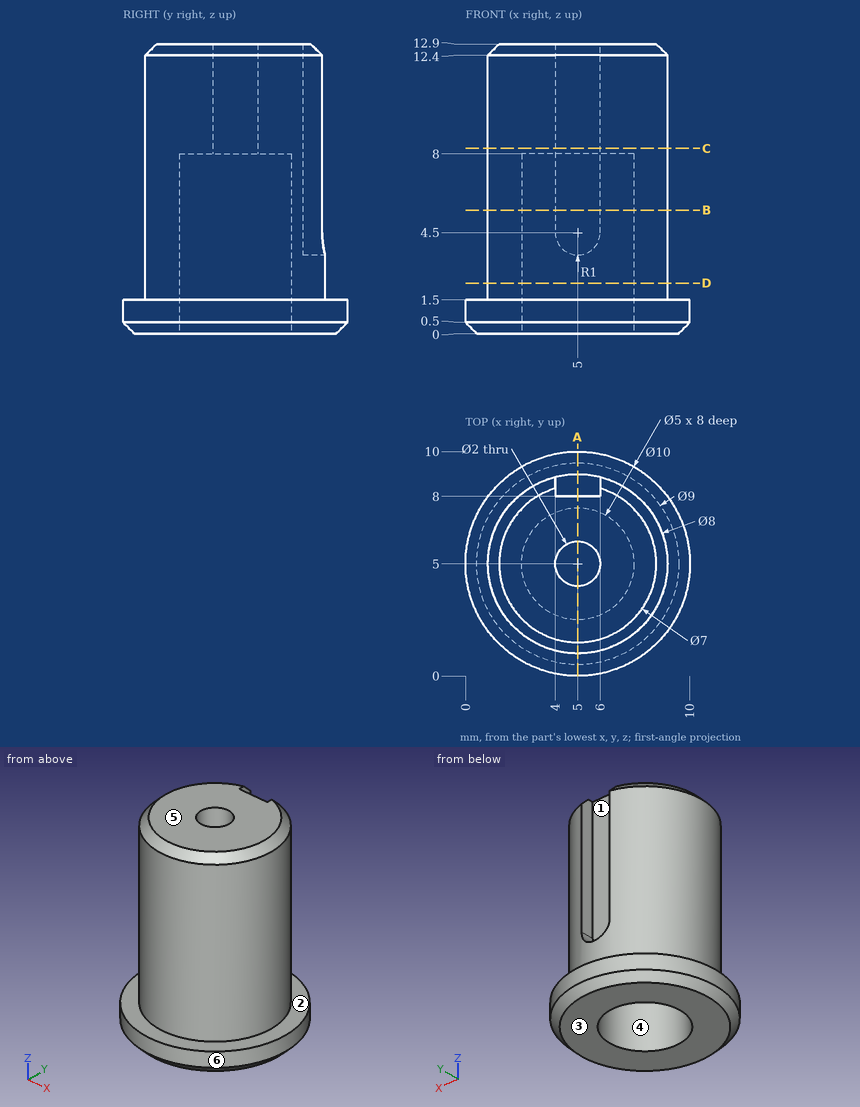
Here's the drawing with two shaded views (mm, measured from the low corner). I have some questions. A direction names the side the tool comes from. Coordinates: 2 decimals unless noted, no trailing zeros. Order: outer loops, then holes, each group sorted by start corner. A loop starts at its lowest first (then second) coordinate and runs counter-clockwise, first axis right, second up. Notation, with made-up numbers: (30, 56) - (51, 56) arc R19 ccw to (51, 88) - close; hole circle Ø2 at (62.5, -23). An arc over 180 degrees is marked (long way). Use CSV: the item, a comma, the result in double quotes. Start each with the question number.
1. Please list where these lines run through material, in increasing order: line 1 (Y direction, x = 5, z = 11.5); line 2 (Y direction, x = 5, z = 5); line 3 (X direction, y = 5, z = 4.5). Write a range as from..to.
2. Suppose I cut it at A-A on x = 5. List the corners of the cut face in (y, z) for me.
3. Suppose I cut it at C-C on z = 8.25. List the corners of the cut face in (x, y) for me, then the cut area to 3 significant figures.
4. For the marked faces 1, 2 and 3, which set-ups out of +Z, -Z, +X, -X, +Y, -Y let a thin tool reach every point of the face, with its end or its side?
5. I'm going to push flat-ended pins straight in: pin 1 (0.7 mm diameter, centred on y = 8.5, z = 7.5, fed in from -X); pin 2 (0.7 mm diameter, centred on y = 8.5, z = 7.5, fed in from +X); pin 3 (1 mm diameter, centred on y = 5, z = 8, fed in from -X); pin 4 (1.6 mm diameter, centred on x = 5, y = 5, fed in from +Z). Where does each tip first touch, or does it pass through?
6. If we mould it in two halves opening along X, with no side actions, what happens to the marked faces 4, 5 and 6? For each: +X half, -X half, draft (parallel to the pull), parting line (faces both ways), or undercut.
7. Suppose I cut it at D-D on z = 2.25. List the corners of the cut face in (x, y) for me, then the cut area to 3 significant figures.
8. Suppose I cut it at B-B on z = 5.5. List the corners of the cut face in (x, y) for me, then the cut area to 3 significant figures.
Output:
1,line 1,"y = 1..4, 6..8"
1,line 2,"y = 1..2.5, 7.5..8"
1,line 3,"x = 1..2.5, 7.5..9"
2,outline,"(0, 0.5) - (0.5, 0) - (2.5, 0) - (2.5, 8) - (4, 8) - (4, 12.9) - (1.5, 12.9) - (1, 12.4) - (1, 1.5) - (0, 1.5) - close; (6, 8) - (7.5, 8) - (7.5, 0) - (9.5, 0) - (10, 0.5) - (10, 1.5) - (9, 1.5) - (9, 3.5) - (8, 3.5) - (8, 12.9) - (6, 12.9) - close"
3,outline,"(4, 8) - (4, 8.87) arc R4 ccw (long way) to (6, 8.87) - (6, 8) - close; hole circle Ø2 at (5, 5)"
3,area,"45.2 mm2"
4,face 1,"+Z, +Y"
4,face 2,"+Z"
4,face 3,"-Z, +X, -X, +Y, -Y"
5,pin 1,"stops at x = 2.53"
5,pin 2,"stops at x = 7.47"
5,pin 3,"stops at x = 1"
5,pin 4,"passes through"
6,face 4,"undercut"
6,face 5,"draft"
6,face 6,"parting line"
7,outline,"circle Ø8 at (5, 5); hole circle Ø5 at (5, 5)"
7,area,"30.6 mm2"
8,outline,"(4, 8) - (4, 8.87) arc R4 ccw (long way) to (6, 8.87) - (6, 8) - close; hole circle Ø5 at (5, 5)"
8,area,"28.7 mm2"
